Design review of the part built by this model. Coordinates are the model's own, in mm. Round coordinates to 2 decimals unless told otherwise and drop trailing zeros. Write each loop counter-clockwise with the first axis right and the second up, starting at its lowest first coordinate (ties: lowest second). Pieces come first, ordered by that corner, then holes. Notation, with made-up numbers: (8, 49.5) - (66, 49.5) arc R13 ccw to (66, 59.5) - close; hole circle Ø11 at (32.5, 23.5). An arc over 180 degrees is marked (long way). Use one line per item in the form item = value.
```python
from build123d import *

# Parameters (mm, degrees)
SALIENTE_EXTRUIR1_DEPTH = 25
CROQUIS3_R              = 1.5
CORTAR_EXTRUIR1_DEPTH   = 25
REDONDEO1_R             = 0.5


with BuildPart() as part:
    # Croquis1 → Saliente-Extruir1 (new body)
    with BuildSketch(Plane.XY):
        Polygon((1.178162087, -2.086328696), (2.395894695, -0.022846051), (1.217732608, 2.063482646), (-1.178162087, 2.086328696), (-2.395894695, 0.022846051), (-1.217732608, -2.063482646), align=None)
    extrude(amount=SALIENTE_EXTRUIR1_DEPTH)

    # Croquis3 → Cortar-Extruir1 (cut)
    with BuildSketch(Plane.XY.offset(25)):
        Circle(CROQUIS3_R)
    extrude(amount=-CORTAR_EXTRUIR1_DEPTH, mode=Mode.SUBTRACT)

    # Redondeo1
    redondeo1_edges = [part.edges().sort_by_distance(p)[0] for p in [
        (1.806813652, 1.020318297, 25),
        (-1.217732608, -2.063482646, 12.5),
        (-2.395894695, 0.022846051, 12.5),
        (-1.178162087, 2.086328696, 12.5),
        (1.217732608, 2.063482646, 12.5),
        (2.395894695, -0.022846051, 12.5),
        (1.178162087, -2.086328696, 12.5),
        (0.01978526, 2.074905671, 25),
        (-1.787028391, 1.054587374, 25),
        (-1.806813652, -1.020318297, 25),
        (-0.01978526, -2.074905671, 25),
        (-1.806813652, -1.020318297, 0),
        (-1.787028391, 1.054587374, 0),
        (0.01978526, 2.074905671, 0),
        (1.787028391, -1.054587374, 25),
        (1.806813652, 1.020318297, 0),
        (1.787028391, -1.054587374, 0),
        (-0.01978526, -2.074905671, 0),
    ]]
    fillet(redondeo1_edges, radius=REDONDEO1_R)


solid = part.part
```
Q1. Draft analysis for pull direction X (two halves, no side actions). For faces 1 (the cylindrical face through (-1.5, 0.07, 12.68)), 2 (the cylindrical face through (-1.67, -0.957, 24.857)), 3 (the cylindrical face through (1.676, 0.961, 24.85)), state which applies: released by +X, released by -X, zero draft, split by the parting line, or undercut.
Calculated:
face_1 = undercut
face_2 = released by -X
face_3 = released by +X
Q2. We need section A-A on z = 12.25. Write out the cut boundary in (x, y).
Calculated:
outline = (-2.25, -0.23) - (-1.36, -1.81) arc R0.5 ccw to (-0.93, -2.07) - (0.89, -2.08) arc R0.5 ccw to (1.32, -1.84) - (2.25, -0.27) arc R0.5 ccw to (2.25, 0.23) - (1.36, 1.81) arc R0.5 ccw to (0.93, 2.07) - (-0.89, 2.08) arc R0.5 ccw to (-1.32, 1.84) - (-2.25, 0.27) arc R0.5 ccw to start; hole circle Ø3 at (0, 0)
Q3. For P1, Ø2, axis at x = 0.5, z = 8.5, coming from the +Y side, flat-tipped, find the tip position at first contact; note if it passes through.
Calculated:
P1 = 2.08
Q4. To check wall thickness, follow line 1 along X through (y, z) = (1.3, 1.5); line 2 along Y through (x, z) = (0, 6.25); line 3 along X through (y, z) = (-1.2, 13). State the ranges of each line that lie inside material, in increasing order. Write a range as from..to.
Calculated:
line_1 = -1.64..-0.75, 0.75..1.65
line_2 = -2.08..-1.5, 1.5..2.08
line_3 = -1.71..-0.9, 0.9..1.7
